Geometry check sheet. Reference: the model listing, model coordinates, mm. A direction names the side the tool comes from. Give positions to 0.01 mm unless a question says otherwise; leave off trailing zeros. Write each loop counter-clockwise with the first axis right and the second up, starting at its lowest first coordinate (ties: lowest second). Pieces come first, ordered by that corner, then holes. Notation, with made-up numbers: M 30,16.5 L 89,16.5 A15 ccw 89,29.5 Z; hole C 65,81.25 d3. An arc over 180 degrees is marked long. Write each question's results on one line, items separated by ' | '.
```python
from build123d import *

# Parameters (mm, degrees)
BOSS_EXTRUDE1_DEPTH = 150
BOSS_EXTRUDE2_DEPTH = 0.5
BOSS_EXTRUDE3_START = -0.5
BOSS_EXTRUDE3_DEPTH = 0.5


with BuildPart() as part:
    # Sketch1 → Boss-Extrude1 (new body)
    with BuildSketch(Plane.XY):
        with BuildLine():
            Line((0, 0), (14.838134608, 0))
            ThreePointArc((14.838134608, 0), (16.75155177, 0.380602337), (18.373668514, 1.464466094))
            Line((18.373668514, 1.464466094), (30.543324162, 13.634121742))
            ThreePointArc((30.543324162, 13.634121742), (31.802691096, 15.752289806), (31.897349569, 18.214744029))
            Line((31.897349569, 18.214744029), (28.300052509, 35.045088382))
            ThreePointArc((28.300052509, 35.045088382), (26.554897598, 37.887508322), (23.410493196, 39))
            Line((23.410493196, 39), (4.454734574, 39))
            Line((4.454734574, 39), (4.454734574, 39.5))
            Line((4.454734574, 39.5), (23.410493196, 39.5))
            ThreePointArc((23.410493196, 39.5), (26.869338039, 38.276259154), (28.78900844, 35.14959722))
            Line((28.78900844, 35.14959722), (32.3863055, 18.319252867))
            ThreePointArc((32.3863055, 18.319252867), (32.282181181, 15.610553222), (30.896877552, 13.280568351))
            Line((30.896877552, 13.280568351), (18.727221905, 1.110912703))
            ThreePointArc((18.727221905, 1.110912703), (16.942893486, -0.081337429), (14.838134608, -0.5))
            Line((14.838134608, -0.5), (0, -0.5))
            Line((0, -0.5), (0, 0))
        make_face()
    extrude(amount=-BOSS_EXTRUDE1_DEPTH)

    # Sketch2 → Boss-Extrude2 (add)
    with BuildSketch(Plane(origin=(0, 39.5, 0), x_dir=(1, 0, 0), z_dir=(0, 1, 0))):
        with BuildLine():
            Line((4.454734574, 150), (4.454734574, 153.5))
            ThreePointArc((4.454734574, 153.5), (4.601181183, 153.853553391), (4.954734574, 154))
            Line((4.954734574, 154), (9.954734574, 154))
            ThreePointArc((9.954734574, 154), (10.308287964, 153.853553391), (10.454734574, 153.5))
            Line((10.454734574, 153.5), (10.454734574, 150))
            Line((10.454734574, 150), (4.454734574, 150))
        make_face()
        with BuildLine():
            Line((4.454734574, 0), (10.454734574, 0))
            Line((10.454734574, 0), (10.454734574, -3.5))
            ThreePointArc((10.454734574, -3.5), (10.308287964, -3.853553391), (9.954734574, -4))
            Line((9.954734574, -4), (4.954734574, -4))
            ThreePointArc((4.954734574, -4), (4.601181183, -3.853553391), (4.454734574, -3.5))
            Line((4.454734574, -3.5), (4.454734574, 0))
        make_face()
    extrude(amount=-BOSS_EXTRUDE2_DEPTH)

    # Sketch3 → Boss-Extrude3 (add)
    with BuildSketch(Plane.XZ.offset(0.5).offset(BOSS_EXTRUDE3_START)):
        with BuildLine():
            Line((10.454734574, -150), (4.454734574, -150))
            Line((4.454734574, -150), (4.454734574, -153.5))
            ThreePointArc((4.454734574, -153.5), (4.601181183, -153.853553391), (4.954734574, -154))
            Line((4.954734574, -154), (9.954734574, -154))
            ThreePointArc((9.954734574, -154), (10.308287964, -153.853553391), (10.454734574, -153.5))
            Line((10.454734574, -153.5), (10.454734574, -150))
        make_face()
        with BuildLine():
            Line((10.454734574, 0), (10.454734574, 3.5))
            ThreePointArc((10.454734574, 3.5), (10.308287964, 3.853553391), (9.954734574, 4))
            Line((9.954734574, 4), (4.954734574, 4))
            ThreePointArc((4.954734574, 4), (4.601181183, 3.853553391), (4.454734574, 3.5))
            Line((4.454734574, 3.5), (4.454734574, 0))
            Line((4.454734574, 0), (10.454734574, 0))
        make_face()
    extrude(amount=BOSS_EXTRUDE3_DEPTH)


solid = part.part
```
Q1. Section check D-D (y = 29). Enter the section's corners in (x, z).
Answer key:
outline: M 29.59,-150 L 30.1,-150 L 30.1,0 L 29.59,0 Z
Q2. Material ranges on probe 1 along Y at (x, z) = (10.5, -2.5); probe 2 along Y at (x, z) = (22.5, -127); probe 3 along X at (y, z) = (6, -136.5), recorded low to high. Write a range as [from, to].
Answer key:
probe 1: y = [-0.5, 0], [39, 39.5] | probe 2: y = [4.88, 5.59], [39, 39.5] | probe 3: x = [22.91, 23.62]
Q3. Depth check by flat-ended pin: P1, Ø6, axis at x = 26.5, z = -110.5, coming from the -Y side; P2, Ø6, axis at y = 26.5, z = -81.5, coming from the -X side; P3, Ø0.6, axis at y = -0.5, z = 1.5, coming from the -X side; P4, Ø5, axis at x = 11, y = 3.5, coming from the +Z side. Enter the tip coordinate at first touch or a pass-through.
Answer key:
P1: stops at y = 5.88 | P2: stops at x = 29.49 | P3: stops at x = 4.45 | P4: passes through
Q4. Section check A-A (x = 7). Enter the section's corners in (y, z).
Answer key:
outline: M -0.5,-154 L 0,-154 L 0,4 L -0.5,4 Z; M 39,-154 L 39.5,-154 L 39.5,4 L 39,4 Z
Q5. Section check B-B (z = -92.5). Enter the section's corners in (x, y).
Answer key:
outline: M 0,-0.5 L 14.84,-0.5 A5.5 ccw 18.73,1.11 L 30.9,13.28 A5.5 ccw 32.39,18.32 L 28.79,35.15 A5.5 ccw 23.41,39.5 L 4.45,39.5 L 4.45,39 L 23.41,39 A5 cw 28.3,35.05 L 31.9,18.21 A5 cw 30.54,13.63 L 18.37,1.46 A5 cw 14.84,0 L 0,0 Z
Q6. Release check for a two-part mould opening along Y. For faces 1 (the face through (30.124, 26.512, -73.95)), 2 (the face through (30.562, 26.852, -73.95)), 3 (the face through (16.97, -0.07, -73.95)) record: released by +Y, released by -Y, zero draft, split by the parting line, or undercut.
Answer key:
face 1: undercut | face 2: released by +Y | face 3: released by -Y
Q7. Access from +Z, -Z, +X, -X, +Y, -Y to the whole of each face (thin tool, end or side, straight path). Record for faces 4 (the face through (32.293, 15.647, -73.95)), 5 (the face through (26.59, 37.86, -73.95)).
Answer key:
face 4: +Z, -Z, +X | face 5: +Z, -Z, -X
Q8. Section check C-C (x = 13.5). Enter the section's corners in (y, z), then the cut area to 3 significant figures.
Answer key:
outline: M -0.5,-150 L 0,-150 L 0,0 L -0.5,0 Z; M 39,-150 L 39.5,-150 L 39.5,0 L 39,0 Z | area: 150 mm2
